The model under review builds one solid part; all positions refer to its coordinate system, in mm. A direction names the side the tool comes from. Round coordinates to 2 decimals unless told otherwise and drop trailing zeros. Loops run counter-clockwise (first coordinate to the right, second up) from the corner with the lowest first, then second, coordinate; pieces in that order, holes last. Notation, with made-up numbers: (4, 85.25) -> (55, 85.25) arc R26 cw to (55, 111.25) -> close; hole circle Ø4 at (61, 46.5). An arc over 180 degrees is marked (long way). Use a Markdown table: item, result. Add a question column.
1) Insertion check: pin 1 (10 mm diameter, centred on y = -18, z = 9.5, fed in from -X); pin 2 (2 mm diameter, centred on x = 22, z = 10, fed in from +Y); pin 3 (6 mm diameter, centred on y = -29.5, z = 10, fed in from +X). Each pin has a flat end and moves straight along its axis. Give the tip position at first contact, or say it passes through.
2) Mouldability with a two-part tool opening along Z and no side actions: class faces 5 (the flat face through (20, -18, 0)), 6 (the flat face through (30, 6.6, 10)), 7 (the cylindrical face through (-0.9, -8.5, 15.2)), 8 (the flat face through (20, -18, 20)) as released by +Z, released by -Z, zero draft, split by the parting line, or undercut.
3) Wall thickness on probe 1 along Z at (x, y) = (43.9, -9.2); probe 2 along X at (y, z) = (-2, 10.5); probe 3 along Y at (x, z) = (28, 7.5): over which ranges is each line inside the solid? List them lowest first.
4) Consider section B-B on z = 15.1. Give the boundary of the cut face in (x, y), plus the area to 3 significant figures.
5) Consider section C-C on x = 30. Give the boundary of the cut face in (y, z), plus the area to 3 significant figures.
6) For faces 1 (the flat face through (40, -23, 10)), 2 (the flat face through (-2, -7, 10)), 3 (the flat face through (43, -7, 10)), 4 (the cylindrical face through (27.3, 3.3, 9.9)), list the 3-axis set-ups (+Z, -Z, +X, -X, +Y, -Y) from which the entire face can be reached by the end or side of a thin tool; tool diameter is ignored.
7) Consider section A-A on x = 43.9. Give the boundary of the cut face in (y, z).
8) Consider section D-D on y = -13.5. Give the boundary of the cut face in (x, z), plus the area to 3 significant figures.
from build123d import *

# Parameters (mm, degrees)
EXTRUDE_1_DEPTH     = 20
SKETCH_2_R          = 3
CUT_EXTRUDE_1_DEPTH = 30.5
SKETCH_3_R          = 2.7
EXTRUDE_2_DEPTH     = 6.6


with BuildPart() as part:
    # 草圖1 → 填料-伸長1 (new body)
    with BuildSketch(Plane.XY):
        Polygon((0, -7), (-6.4, -7), (-6.4, -10), (0, -10), (0, -36.5), (40, -36.5), (40, -10), (46.4, -10), (46.4, -7), (40, -7), (40, 0), (0, 0), align=None)
    extrude(amount=EXTRUDE_1_DEPTH)

    # 草圖2 → 除料-伸長1 (cut, through all)
    with BuildSketch(Plane(origin=(0, -7, 0), x_dir=(1, 0, 0), z_dir=(0, 1, 0))):
        with Locations((-3.9, -4.9)):
            Circle(SKETCH_2_R)
        with Locations((-3.9, -15.1)):
            Circle(SKETCH_2_R)
        with Locations((43.9, -15.1)):
            Circle(SKETCH_2_R)
        with Locations((43.9, -4.9)):
            Circle(SKETCH_2_R)
    extrude(amount=-CUT_EXTRUDE_1_DEPTH, mode=Mode.SUBTRACT)

    # 草圖3 → 填料-伸長2 (add)
    with BuildSketch(Plane(origin=(0, 0, 0), x_dir=(1, 0, 0), z_dir=(0, 1, 0))):
        with Locations((30, -10)):
            Circle(SKETCH_3_R)
    extrude(amount=EXTRUDE_2_DEPTH)


solid = part.part
Result set:
| question | item | result |
|---|---|---|
| 1 | pin 1 | x = 0 |
| 1 | pin 2 | y = 0 |
| 1 | pin 3 | x = 40 |
| 2 | face 5 | released by -Z |
| 2 | face 6 | zero draft |
| 2 | face 7 | undercut |
| 2 | face 8 | released by +Z |
| 3 | probe 1 | 0 to 1.9, 7.9 to 12.1, 18.1 to 20 |
| 3 | probe 2 | 0 to 40 |
| 3 | probe 3 | -36.5 to 0 |
| 4 | outline | (-0.9, -10) -> (0, -10) -> (0, -36.5) -> (40, -36.5) -> (40, -10) -> (40.9, -10) -> (40.9, -7) -> (40, -7) -> (40, 0) -> (0, 0) -> (0, -7) -> (-0.9, -7) -> close |
| 4 | area | 1,470 mm2 |
| 5 | outline | (-36.5, 0) -> (0, 0) -> (0, 7.3) -> (6.6, 7.3) -> (6.6, 12.7) -> (0, 12.7) -> (0, 20) -> (-36.5, 20) -> close |
| 5 | area | 766 mm2 |
| 6 | face 1 | +Z, -Z, +X, -Y |
| 6 | face 2 | +Z, -Z, -X, +Y |
| 6 | face 3 | +Z, -Z, +X, +Y |
| 6 | face 4 | +Y |
| 7 | outline | (-10, 0) -> (-7, 0) -> (-7, 1.9) -> (-10, 1.9) -> close; (-10, 7.9) -> (-7, 7.9) -> (-7, 12.1) -> (-10, 12.1) -> close; (-10, 18.1) -> (-7, 18.1) -> (-7, 20) -> (-10, 20) -> close |
| 8 | outline | (0, 0) -> (40, 0) -> (40, 20) -> (0, 20) -> close |
| 8 | area | 800 mm2 |
